from build123d import *

# Parameters (mm, degrees)
F0_W     = 15
F0_H     = 7.9
F0_R     = 2.95
F1_DEPTH = 8
F0_R_2   = 0.75
F2_DEPTH = 1


with BuildPart() as f1:
    # F0 (on Top) → F1 (new body)
    with BuildSketch(Plane.XY):
        with Locations((7.5, 3.95)):
            Rectangle(F0_W, F0_H)
        with Locations((7.5, 3.95)):
            Circle(F0_R, mode=Mode.SUBTRACT)
    extrude(amount=F1_DEPTH)

    # F0 (on Top) → F2 (join)
    with BuildSketch(Plane.XY):
        with Locations((7.5, 3.95)):
            Circle(F0_R)
        with Locations((7.5, 3.95)):
            Circle(F0_R_2, mode=Mode.SUBTRACT)
    extrude(amount=F2_DEPTH)


solid = f1.part
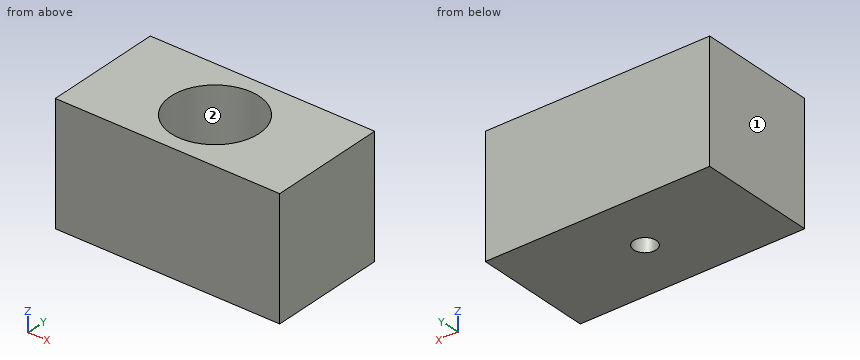
The listing builds one solid part. Answer for the finished solid, in the listing's coordinates (mm). Face numbers are marked on the shaded views. A direction names the side the tool comes from. Round coordinates to 2 decimals unless told otherwise and drop trailing zeros. Order: outer loops, then holes, each group sorted by start corner. A loop starts at its lowest first (then second) coordinate and runs counter-clockwise, first axis right, second up. Notation, with made-up numbers: M 24,62.5 L 83,62.5 A23 cw 83,90.5 Z; hole C 25.25,2.5 d10. An arc over 180 degrees is marked long. Answer in a Markdown table with one row per item. Add a question column.
1) Which of the six approach directions +Z, -Z, +X, -X, +Y, -Y give full straight-line access (tool end or side, diameter ignored) to the marked faces 1 and 2?
2) Consider line 1 along Y through (x, z) = (7.5, 3.5); line 2 along Y through (x, z) = (7.5, 0.5); line 3 along X through (y, z) = (6.25, 4). Determine where each line is inside the solid, lowest interval first. Write a range as from..to.
3) The part is cut by section B-B on y = 3.95. Determine the outline of the cut face in (x, z), plus the area to 3 significant figures.
4) The part is cut by section C-C on z = 3.5. Determine the outline of the cut face in (x, y), plus the area to 3 significant figures.
5) The part is cut by section D-D on y = 3. Determine the outline of the cut face in (x, z).
6) Flat-ended cylindrical pins translate along their axes: pin 1 Ø1.4 at (x, y) = (7.5, 3.95) entering from +Z; pin 2 Ø1.8 at (x, y) = (8.5, 4.5) entering from +Z. Find the tip coordinate at first contact, or state that the pin passes through.
7) The part is cut by section A-A on x = 7.5. Determine the outline of the cut face in (y, z).
Findings below:
| question | item | result |
|---|---|---|
| 1 | face 1 | +Z, -Z, -X, +Y, -Y |
| 1 | face 2 | +Z |
| 2 | line 1 | y = 0..1, 6.9..7.9 |
| 2 | line 2 | y = 0..3.2, 4.7..7.9 |
| 2 | line 3 | x = 0..5.65, 9.35..15 |
| 3 | outline | M 0,0 L 6.75,0 L 6.75,1 L 4.55,1 L 4.55,8 L 0,8 Z; M 8.25,0 L 15,0 L 15,8 L 10.45,8 L 10.45,1 L 8.25,1 Z |
| 3 | area | 77.2 mm² |
| 4 | outline | M 0,0 L 15,0 L 15,7.9 L 0,7.9 Z; hole C 7.5,3.95 d5.9 |
| 4 | area | 91.2 mm² |
| 5 | outline | M 0,0 L 15,0 L 15,8 L 10.29,8 L 10.29,1 L 4.71,1 L 4.71,8 L 0,8 Z |
| 6 | pin 1 | passes through |
| 6 | pin 2 | stops at z = 1 |
| 7 | outline | M 0,0 L 3.2,0 L 3.2,1 L 1,1 L 1,8 L 0,8 Z; M 4.7,0 L 7.9,0 L 7.9,8 L 6.9,8 L 6.9,1 L 4.7,1 Z |
